CAD build for the part. Positions are in the model's coordinates, mm. A direction names the side the tool comes from. Round coordinates to 2 decimals unless told otherwise and drop trailing zeros. Loops run counter-clockwise (first coordinate to the right, second up) from the corner with the lowest first, then second, coordinate; pieces in that order, holes last. Notation, with made-up numbers: M 7,-17 L 17,-17 A36 cw 17,17 Z; hole C 77,22.25 d11. An arc over 180 degrees is marked long. Use one line per item in the form item = value.
from build123d import *

# Parameters (mm, degrees)
SKETCH1_R           = 21
BOSS_EXTRUDE1_DEPTH = 2
SKETCH2_R           = 20
BOSS_EXTRUDE2_DEPTH = 46
SKETCH3_R           = 12.5
CUT_EXTRUDE1_DEPTH  = 49
SKETCH4_W           = 8
SKETCH4_H           = 7
CUT_EXTRUDE2_DEPTH  = 48


with BuildPart() as part:
    # Sketch1 → Boss-Extrude1 (new body)
    with BuildSketch(Plane.XY):
        Circle(SKETCH1_R)
    extrude(amount=BOSS_EXTRUDE1_DEPTH)

    # Sketch2 → Boss-Extrude2 (add)
    with BuildSketch(Plane.XY.offset(2)):
        Circle(SKETCH2_R)
    extrude(amount=BOSS_EXTRUDE2_DEPTH)

    # Sketch3 → Cut-Extrude1 (cut, through all)
    with BuildSketch(Plane(origin=(0, 0, 0), x_dir=(-1, 0, 0), z_dir=(0, 0, -1))):
        Circle(SKETCH3_R)
    extrude(amount=-CUT_EXTRUDE1_DEPTH, mode=Mode.SUBTRACT)

    # Sketch4 → Cut-Extrude2 (cut)
    with BuildSketch(Plane(origin=(0, 0, 0), x_dir=(-1, 0, 0), z_dir=(0, 0, -1))):
        with Locations((0, 12.5)):
            Rectangle(SKETCH4_W, SKETCH4_H)
    extrude(amount=-CUT_EXTRUDE2_DEPTH, mode=Mode.SUBTRACT)


solid = part.part
1. Cut at A-A on x = 0. Write the cut outline in (y, z).
Completed:
outline = M -21,0 L -12.5,0 L -12.5,48 L -20,48 L -20,2 L -21,2 Z; M 16,0 L 21,0 L 21,2 L 20,2 L 20,48 L 16,48 Z
2. Cut at B-B on y = 0. Write the cut outline in (x, z), and give its area (3 significant figures).
Completed:
outline = M -21,0 L -12.5,0 L -12.5,48 L -20,48 L -20,2 L -21,2 Z; M 12.5,0 L 21,0 L 21,2 L 20,2 L 20,48 L 12.5,48 Z
area = 724 mm2
3. Cut at C-C on z = 13.5. Write the cut outline in (x, y), and give its area (3 significant figures).
Completed:
outline = C 0,0 d40; hole M -4,11.84 A12.5 ccw long 4,11.84 L 4,16 L -4,16 Z
area = 736 mm2
4. Pull direction Y, two halves, no side cores. Call faces 4 (the face through (19, -8, 2)), 5 (the face through (20.03, 6.31, 0.99)), 6 (the face through (0, 16, 24)): +Y half, -Y half, draft (parallel to the pull), parting line (faces both ways), or undercut.
Completed:
face_4 = draft
face_5 = parting line
face_6 = undercut
5. Tool access for faces 1 (the face through (9, -9, 0)), 2 (the face through (-4.336, -19.524, 24.678)), 3 (the face through (4, 14, 24)): list every direction of +Z, -Z, +X, -X, +Y, -Y with a clear straight run to the whole face (end or side of a thin tool).
Completed:
face_1 = -Z, +X, -X, +Y, -Y
face_2 = +Z
face_3 = +Z, -Z
6. Cut at D-D on y = -14. Write the cut outline in (x, z).
Completed:
outline = M -15.65,0 L 15.65,0 L 15.65,2 L 14.28,2 L 14.28,48 L -14.28,48 L -14.28,2 L -15.65,2 Z
7. Probe line 1 along Y through (x, z) = (-7, 14.5) (3 decimals); line 2 along X through (y, z) = (11, 42); line 3 along Y through (x, z) = (9, 45.5). List the from-to ranges inside material, lowest first. Write a range as from..to.
Completed:
line_1 = -18.735..-10.356, 10.356..18.735
line_2 = -16.7..-5.94, 5.94..16.7
line_3 = -17.86..-8.67, 8.67..17.86
8. Drop flat-ended pins along their axis: P1, Ø2, axis at x = 1, z = 39.5, coming from the +Y side; P2, Ø3, axis at y = -10.5, z = 21, coming from the +X side; P3, Ø10, axis at y = -12, z = 40.5, coming from the -X side (3 decimals); P4, Ø1, axis at x = 11.5, y = -3, coming from the +Z side. Give the stop position or say it passes through.
Completed:
P1 = 20
P2 = 17.86
P3 = -18.735
P4 = through
